Build history of the part. All positions in model axes, mm. A direction names the side the tool comes from. Round coordinates to 2 decimals unless told otherwise and drop trailing zeros. Loops run counter-clockwise (first coordinate to the right, second up) from the corner with the lowest first, then second, coordinate; pieces in that order, holes last. Notation, with made-up numbers: (54, 19.25) -> (108, 19.25) arc R34 ccw to (108, 54.25) -> close; hole circle Ø1 at (65.5, 37). An arc over 180 degrees is marked (long way). Put each result on its own line as item: value. Start each with the question number.
Item 1: Cut at B-B, the plane x = 44. List the corners of the cut face in (y, z), plus the area to 3 significant figures.
Item 2: Tool access for faces 4 (the flat face through (41, 9, 22)), 5 (the flat face through (40.5, 3, 20)), 6 (the flat face through (38, 3, 20)), 7 (the cylindrical face through (43.9, 9.5, 20)), 8 (the flat face through (41, 9, 18)): list every direction of +Z, -Z, +X, -X, +Y, -Y with a clear straight run to the whole face (end or side of a thin tool).
Item 3: Pull direction X, two halves, no side cores. Call faces 1 (the flat face through (-11, -5, 65)), 2 (the flat face through (-55, -5, 0)), 3 (the cylindrical face through (53.986, -5.577, 59.297)): +X half, -X half, draft (parallel to the pull), parting line (faces both ways), or undercut.
Item 4: Flat gauge pins, fed straight in: pin 1 Ø6 at (x, y) = (35.5, 6.5) entering from +Z; pin 2 Ø5 at (y, z) = (-2, -35) entering from +X; pin 3 Ø1.2 at (y, z) = (2.5, 21) entering from +X. Where does each tip first touch, or does it go through?
Item 5: Cut at A-A, the plane y = -6. List the corners of the cut face in (x, z).
Item 6: Cut at C-C, the plane z = 40.5. List the corners of the cut face in (x, y), plus the area to 3 significant figures.
Item 7: Cut at D-D, the plane x = -40.5. List the corners of the cut face in (y, z), plus the area to 4 significant figures.
Item 8: Drill centre lines: probe 1 along X at (y, z) = (-0.5, 6); probe 2 along Y at (x, z) = (40, -7); probe 3 along X at (y, z) = (-3.75, 52) (3 decimals). Where is each one in solid material? Low to high. Write a range as [from, to].
```python
from build123d import *

# Parameters (mm, degrees)
SKETCH2_W           = 140
SKETCH2_H           = 115
BOSS_EXTRUDE1_DEPTH = 11
SKETCH3_W           = 10
SKETCH3_H           = 25
CUT_EXTRUDE1_DEPTH  = 104.662915259
FILLET1_R           = 20
BOSS_EXTRUDE2_DEPTH = 2


with BuildPart() as part:
    # Sketch2 → Boss-Extrude1 (new body)
    with BuildSketch(Plane(origin=(0, 0, 0), x_dir=(1, 0, 0), z_dir=(0, 1, 0))):
        with Locations((-10, -7.5)):
            Rectangle(SKETCH2_W, SKETCH2_H)
    extrude(amount=-BOSS_EXTRUDE1_DEPTH)

    # Sketch3 → Cut-Extrude1 (cut, through all)
    with BuildSketch(Plane(origin=(0, 0, 0), x_dir=(1, 0, 0), z_dir=(0, 1, 0))):
        with Locations((-60, 0)):
            Rectangle(SKETCH3_W, SKETCH3_H)
    extrude(amount=-CUT_EXTRUDE1_DEPTH, mode=Mode.SUBTRACT)

    # Fillet1
    fillet1_edges = [part.edges().sort_by_distance(p)[0] for p in [
        (-80, -5.5, -50),
        (60, -5.5, -50),
        (60, -5.5, 65),
        (-80, -5.5, 65),
    ]]
    fillet(fillet1_edges, radius=FILLET1_R)

    # Sketch4 → Boss-Extrude2 (add, symmetric)
    with BuildSketch(Plane.XY.offset(20)):
        with BuildLine():
            Line((38, 6), (38, 0))
            Line((38, 0), (40.5, 0))
            Line((40.5, 0), (40.5, 6))
            ThreePointArc((40.5, 6), (44, 9.5), (47.5, 6))
            Line((47.5, 6), (50, 6))
            ThreePointArc((50, 6), (44, 12), (38, 6))
        make_face()
    extrude(amount=BOSS_EXTRUDE2_DEPTH, both=True)


solid = part.part
```
Reply:
1. outline: (-11, -49.6) -> (0, -49.6) -> (0, 64.6) -> (-11, 64.6) -> close; (9.5, 18) -> (12, 18) -> (12, 22) -> (9.5, 22) -> close
1. area: 1,270 mm^2
2. face 4: +Z, +X, -X, +Y
2. face 5: +Z, -Z, +X
2. face 6: +Z, -Z, -X, +Y
2. face 7: +Z, -Z
2. face 8: -Z, +X, -X, +Y
3. face 1: draft
3. face 2: undercut
3. face 3: +X half
4. pin 1: stops at z = 22
4. pin 2: stops at x = 59.84
4. pin 3: stops at x = 40.5
5. outline: (-80, -30) arc R20 ccw to (-60, -50) -> (40, -50) arc R20 ccw to (60, -30) -> (60, 45) arc R20 ccw to (40, 65) -> (-60, 65) arc R20 ccw to (-80, 45) -> close; hole (-65, -12.5) -> (-55, -12.5) -> (-55, 12.5) -> (-65, 12.5) -> close
6. outline: (-80, -11) -> (60, -11) -> (60, 0) -> (-80, 0) -> close
6. area: 1,540 mm^2
7. outline: (-11, -50) -> (0, -50) -> (0, 65) -> (-11, 65) -> close
7. area: 1,265 mm^2
8. probe 1: x = [-80, -65], [-55, 60]
8. probe 2: y = [-11, 0]
8. probe 3: x = [-78.735, 58.735]
